Autodesk Fusion 360 part; units mm, degrees
sketch "Schizzo1" plane through (0, 0, 0) normal (0, 0, 1) x (1, 0, 0)
  line L0 (39.1195, 62.1228) -> (89.1195, 62.1228)
  line L1 (89.1195, 62.1228) -> (89.1195, 12.5228)
  line L2 (89.1195, 12.5228) -> (39.1195, 12.5228)
  line L3 (39.1195, 12.5228) -> (39.1195, 62.1228)
  line L4 (43.6195, 62.1228) -> (43.6195, 12.5228)
  line L5 (74.1195, 62.1228) -> (74.1195, 12.5228)
  line L6 (39.1195, 37.3228) -> (89.1195, 37.3228) construction
  line L7 (48.1195, 62.1228) -> (48.1195, 12.5228) construction
  circle A0 centre (48.1195, 57.6228) radius 2.5
  circle A1 centre (48.1195, 17.0228) radius 2.5
  line L8 (74.1195, 37.3228) -> (89.1195, 37.3228)
  line L9 (86.071, 62.1228) -> (86.071, 12.5228) construction
  line L10 (59.1195, 62.1228) -> (59.1195, 37.3228)
  line L11 (74.1195, 37.3228) -> (59.1195, 37.3228)
  line L12 (39.1195, 52.3228) -> (43.6195, 52.3228)
  line L13 (43.6195, 52.3228) -> (43.6195, 47.3228)
  line L14 (43.6195, 47.3228) -> (39.1195, 47.3228)
  line L15 (39.1195, 47.3228) -> (39.1195, 52.3228)
  line L16 (43.6195, 27.3228) -> (39.1195, 27.3228)
  line L17 (39.1195, 22.3228) -> (43.6195, 22.3228)
  line L18 (39.1195, 49.8228) -> (43.6195, 49.8228) construction
  line L19 (39.1195, 24.8228) -> (43.6195, 24.8228) construction
  dimension "d1" = 50
  dimension "d2" = 49.6
  dimension "d3" = 4.5
  dimension "d4" = 15
  dimension "d6" = 5
  dimension "d7" = 40.6
  dimension "d26" = 9
  dimension "d29" = 15
  dimension "d40" = 5
  dimension "d41" = 25
extrude "Estrusione1" add sketch "Schizzo1" along normal blind 3 contours L0 L2 L4 L5 L10 L11 L13
extrude "Estrusione7" add sketch "Schizzo1" along normal blind 2 contours L0 L5 L10 L11
extrude "Estrusione2" add sketch "Schizzo1" along normal blind 0.4 contours L1 L2 L5 L8
extrude "Estrusione6" add sketch "Schizzo1" along normal blind 1 contours L0 L1 L5 L8
extrude "Estrusione3" add sketch "Schizzo1" along normal blind 1.5 contours L0 L3 L4 L12 | L3 L4 L14 L16 | L2 L3 L4 L17
sketch "Schizzo4" plane through (0, 0, 3) normal (0, 0, 1) x (-1, 0, 0)
  circle A0 centre (-48.1195, -57.6228) radius 2.5
  circle A1 centre (-48.1195, -17.0228) radius 2.5
  line L0 (-74.1195, -12.5228) -> (-74.1195, -37.3228)
  line L1 (-74.1195, -37.3228) -> (-59.1195, -37.3228)
  line L2 (-59.1195, -37.3228) -> (-59.1195, -62.1228)
  line L3 (-59.1195, -62.1228) -> (-43.6195, -62.1228)
  line L4 (-43.6195, -62.1228) -> (-43.6195, -12.5228)
  line L5 (-43.6195, -12.5228) -> (-74.1195, -12.5228)
  line L6 (-59.1195, -37.3228) -> (-45.6195, -37.3228) construction
  line L7 (-51.7809, -60.1228) -> (-57.1195, -60.1228)
  line L8 (-57.1195, -60.1228) -> (-57.1195, -35)
  line L9 (-57.1195, -35) -> (-72.1195, -35)
  line L10 (-72.1195, -35) -> (-72.1195, -14.5228)
  line L11 (-72.1195, -14.5228) -> (-51.7809, -14.5228)
  line L12 (-51.7809, -14.5228) -> (-51.7809, -20.8228)
  line L13 (-51.7809, -20.8228) -> (-45.6195, -20.8228)
  line L14 (-45.6195, -20.8228) -> (-45.6195, -53.8228)
  line L15 (-45.6195, -53.8228) -> (-51.7809, -53.8228)
  line L16 (-51.7809, -53.8228) -> (-51.7809, -60.1228)
  point P0 (-45.6195, -37.3228)
  dimension "d47" = 2
  dimension "d48" = 2
  dimension "d49" = 2
  dimension "d50" = 2
  dimension "d51" = 2
  dimension "d52" = 33
sketch "Schizzo5" plane through (0, 0, 2) normal (0, 0, 1) x (-1, 0, 0)
  line L0 (-59.1195, -62.1228) -> (-59.1195, -37.3228)
  line L1 (-59.1195, -37.3228) -> (-74.1195, -37.3228)
  line L2 (-74.1195, -37.3228) -> (-74.1195, -62.1228)
  line L3 (-74.1195, -62.1228) -> (-59.1195, -62.1228)
  line L4 (-61.1195, -60.1228) -> (-72.1195, -60.1228)
  line L5 (-72.1195, -60.1228) -> (-72.1195, -38.4568)
  line L6 (-72.1195, -38.4568) -> (-61.1195, -38.4568)
  line L7 (-61.1195, -38.4568) -> (-61.1195, -60.1228)
  line L8 (-59.1195, -37.3228) -> (-59.1195, -62.1228)
  dimension "d42" = 2
  dimension "d43" = 2
  dimension "d44" = 2
sketch "Schizzo6" plane through (0, 0, 1) normal (0, 0, 1) x (-1, 0, 0)
  line L0 (-74.1195, -62.1228) -> (-74.1195, -37.3228)
  line L1 (-74.1195, -37.3228) -> (-89.1195, -37.3228)
  line L2 (-89.1195, -37.3228) -> (-89.1195, -62.1228)
  line L3 (-89.1195, -62.1228) -> (-74.1195, -62.1228)
extrude "Estrusione10" cut sketch "Schizzo5" against normal blind 1 contours L4 L5 L6 L7
extrude "Estrusione11" cut sketch "Schizzo4" against normal blind 2 contours L7 L8 L9 L10 L11 L12 L13 L14 L15 L16
extrude "Estrusione9" [suppressed]
extrude "Estrusione8" [suppressed]
equation "d2 = 50 mm - 0.4 mm"
equation "d7 = d2 - 9 mm"
Work out the finished part from the listing and answer in its coordinate system (mm). A direction names the side the tool comes from. Round coordinates to 2 decimals unless told otherwise and drop trailing zeros. Loops run counter-clockwise (first coordinate to the right, second up) from the corner with the lowest first, then second, coordinate; pieces in that order, holes last.
(1) The part is cut by section D-D, the plane y = 56. Give the vertices of the cut face in (x, z).
Computed values:
outline: (39.12, 0) - (46.22, 0) - (46.22, 3) - (43.62, 3) - (43.62, 1.5) - (39.12, 1.5) - close; (50.02, 0) - (89.12, 0) - (89.12, 1) - (74.12, 1) - (74.12, 2) - (72.12, 2) - (72.12, 1) - (61.12, 1) - (61.12, 2) - (59.12, 2) - (59.12, 3) - (57.12, 3) - (57.12, 1) - (51.78, 1) - (51.78, 3) - (50.02, 3) - close
(2) The part is cut by section A-A, the plane x = 43. Give the vertices of the cut face in (y, z), and give its area (3 significant figures).
Computed values:
outline: (12.52, 0) - (22.32, 0) - (22.32, 1.5) - (12.52, 1.5) - close; (27.32, 0) - (47.32, 0) - (47.32, 1.5) - (27.32, 1.5) - close; (52.32, 0) - (62.12, 0) - (62.12, 1.5) - (52.32, 1.5) - close
area: 59.4 mm2
(3) The part is cut by section B-B, the plane y = 43. Give the vertices of the cut face in (x, z), and give its area (4 significant figures).
Computed values:
outline: (39.12, 0) - (89.12, 0) - (89.12, 1) - (74.12, 1) - (74.12, 2) - (72.12, 2) - (72.12, 1) - (61.12, 1) - (61.12, 2) - (59.12, 2) - (59.12, 3) - (57.12, 3) - (57.12, 1) - (45.62, 1) - (45.62, 3) - (43.62, 3) - (43.62, 1.5) - (39.12, 1.5) - close
area: 64.25 mm2
(4) For faces 1 (the flat face through (82, 50, 1)), 2 (the flat face through (41, 47.323, 1)), 3 (the flat face through (51.781, 18, 2)), 4 (the flat face through (41, 37, 1.5)), determine the directions among +Z, -Z, +X, -X, +Y, -Y from which every point of the face is accessible in a straight line to the end or side of a thin tool.
Computed values:
face 1: +Z, +X, +Y, -Y
face 2: +Z, -Z, -X
face 3: +Z
face 4: +Z, -X, +Y, -Y
(5) The part is cut by section C-C, the plane x = 64. Give the vertices of the cut face in (y, z).
Computed values:
outline: (12.52, 0) - (62.12, 0) - (62.12, 2) - (60.12, 2) - (60.12, 1) - (38.46, 1) - (38.46, 2) - (37.32, 2) - (37.32, 3) - (35, 3) - (35, 1) - (14.52, 1) - (14.52, 3) - (12.52, 3) - close
(6) Each of these flat-tipped pins is pushed along its axis until it touches: P1, Ø2, axis at x = 42, y = 59.5, coming from the +Z side; P2, Ø1, axis at y = 51.5, z = 2, coming from the -X side; P3, Ø1, axis at y = 57.5, z = 2, coming from the +X side; P4, Ø4, axis at x = 48.12, y = 17.02, coming from the +Z side. Where does it stop, or does it pass through?
Computed values:
P1: stops at z = 1.5
P2: stops at x = 43.62
P3: stops at x = 74.12
P4: passes through
(7) Find the intervals of material crossed by L1, parallel to Y at x = 67, z = 1.25; L2, parallel to X at y = 21, z = 1.65; L3, parallel to X at y = 45, z = 2.3, in increasing order.
Computed values:
L1: y = 12.52 to 14.52, 35 to 38.46, 60.12 to 62.12
L2: x = 43.62 to 45.62, 72.12 to 74.12
L3: x = 43.62 to 45.62, 57.12 to 59.12
(8) The mould has two halves that part along Y. Classify faces 5 (the flat face through (58, 62.123, 1)), 6 (the flat face through (82, 25, 0.4)), 7 (the cylindrical face through (45.622, 16.913, 1.479)): pulls with the +Y half, pulls with the -Y half, needs draft (parallel to the pull), parting line crosses it, or undercut.
Computed values:
face 5: pulls with the +Y half
face 6: needs draft
face 7: undercut
